Work out the finished part from the listing and answer in its coordinate system (mm). A direction names the side the tool comes from. Give positions to 0.01 mm unless a question says otherwise; leave off trailing zeros. Write each loop counter-clockwise with the first axis right and the second up, starting at its lowest first coordinate (ties: lowest second). Pieces come first, ordered by that corner, then holes. Notation, with made-up numbers: (8.25, 19) - (50.25, 19) arc R18 cw to (50.25, 27) - close; hole circle Ø2 at (68.25, -7). An arc over 180 degrees is marked (long way). Write item = value, one per line.
Autodesk Inventor part; units mm, degrees
ref_plane "YZ Plane" through (0, 0, 0) normal (1, 0, 0) x (0, 1, 0)
ref_plane "XZ Plane" through (0, 0, 0) normal (0, 1, 0) x (-1, 0, 0)
ref_plane "XY Plane" through (0, 0, 0) normal (0, 0, 1) x (1, 0, 0)
sketch "Szkic2" plane through (0, 0, 0) normal (0, 1, 0) x (-1, 0, 0)
  line L0 (10, 40) -> (-10, 40)
  line L1 (-10, 40) -> (-10, -40)
  line L2 (-10, -40) -> (10, -40)
  line L3 (10, -40) -> (10, 40)
  line L4 (10, 40) -> (-10, -40) construction
  line L5 (-10, 40) -> (10, -40) construction
  line L6 (8.6, 38.6) -> (-8.6, 38.6)
  line L7 (-8.6, 38.6) -> (-8.6, -38.6)
  line L8 (-8.6, -38.6) -> (8.6, -38.6)
  line L9 (8.6, -38.6) -> (8.6, 38.6)
  line L10 (8.6, 38.6) -> (-8.6, -38.6) construction
  line L11 (-8.6, 38.6) -> (8.6, -38.6) construction
  point P0 (0, 0)
  point P1 (0, -40)
  dimension "d14" = 20
  dimension "d15" = 80
  dimension "d16" = 1.4
  dimension "d17" = 1.4
extrude "Wyciągnięcie proste2" add sketch "Szkic2" along normal blind 500
sketch "Szkic3" plane through (-10, 0, -40) normal (-1, 0, 0) x (0, 0, 1)
  circle A0 centre (40, 229) radius 2.25
  circle A1 centre (40, 271) radius 2.25
  line L0 (0, 0) -> (0, 500)
  line L1 (0, 500) -> (80, 500)
  point P0 (40, 0)
  point P1 (40, 250)
  point P2 (40, 500)
  dimension "d20" = 4.5
  dimension "d21" = 4.5
  dimension "d22" = 21
  dimension "d23" = 21
  dimension "d24" = 40
  dimension "d25" = 40
  dimension "d26" = 40
  dimension "d27" = 250
extrude "Wyciągnięcie proste3" cut sketch "Szkic3" against normal blind 20
sketch "Szkic4" plane through (-10, 0, -40) normal (-1, 0, 0) x (0, 0, 1)
  point P0 (40, 0)
sketch "Szkic5" plane through (10, 0, 40) normal (1, 0, 0) x (0, 0, -1)
  point P0 (40, 0)
sketch "Szkic6" plane through (10, 0, 40) normal (1, 0, 0) x (0, 0, -1)
  point P0 (40, 0)
sketch "Szkic7" plane through (10, 0, 40) normal (1, 0, 0) x (0, 0, -1)
  line L0 (80, 0) -> (80, 500)
  line L1 (80, 250) -> (0, 250)
  line L2 (1.4, 0) -> (1.4, 500)
  line L3 (80, 250) -> (160, 250) construction
  line L4 (50, 355) -> (30, 355)
  line L5 (30, 355) -> (30, 325)
  line L6 (30, 325) -> (50, 325)
  line L7 (50, 325) -> (50, 355)
  line L8 (50, 355) -> (30, 325) construction
  line L9 (30, 355) -> (50, 325) construction
  line L10 (50, 145) -> (30, 145)
  line L11 (30, 145) -> (30, 175)
  line L12 (30, 175) -> (50, 175)
  line L13 (50, 175) -> (50, 145)
  point P0 (40, 0)
  point P1 (40, 340)
  dimension "d30" = 80
  dimension "d31" = 180
  dimension "d32" = 20
  dimension "d33" = 30
  dimension "d34" = 90
  dimension "d35" = 40
extrude "Wyciągnięcie proste4" cut sketch "Szkic7" against normal blind 1.4
sketch "Szkic8" plane through (-10, 0, -40) normal (-1, 0, 0) x (0, 0, 1)
  line L0 (0, 0) -> (0, 500)
  line L1 (0, 250) -> (80, 250)
  line L2 (80, 0) -> (80, 500)
  line L3 (0, 250) -> (80, 250) construction
  circle A0 centre (40, 40) radius 10
  line L4 (0, 0) -> (80, 0)
  circle A1 centre (40, 460) radius 10
  point P0 (40, 0)
  point P1 (40, 0)
  dimension "d38" = 80
  dimension "d39" = 0
  dimension "d40" = 20
  dimension "d41" = 40
  dimension "d42" = 40
extrude "Wyciągnięcie proste5" cut sketch "Szkic8" against normal blind 1.4 contours A0 | A1
properties part number "belka" material "Aluminium 6061"
1. Find section A-A, the plane z = 31. Give the vertices of the cut face in (x, y).
Solution:
outline = (-10, 0) - (-8.6, 0) - (-8.6, 500) - (-10, 500) - close; (8.6, 0) - (10, 0) - (10, 500) - (8.6, 500) - close
2. A tool of negligible diameter and unlimited length cuts with its end or side. For faces 4 (the flat face through (9, 500, 6)), 5 (the cylindrical face through (-9.31, 469.915, -1.302)), 6 (the flat face through (8.6, 246, 1)), from which of +Z, -Z, +X, -X, +Y, -Y can it reach the whole face along a straight path? Write none if from no direction.
Solution:
face_4 = +Z, -Z, +X, -X, +Y
face_5 = -X
face_6 = +Y, -Y
3. Find section C-C, the plane y = 262. Give the vertices of the cut face in (x, z).
Solution:
outline = (-10, -40) - (10, -40) - (10, 40) - (-10, 40) - close; hole (-8.6, -38.6) - (8.6, -38.6) - (8.6, 38.6) - (-8.6, 38.6) - close
4. Find section B-B, the plane x = -0.75. Give the vertices of the cut face in (y, z), then the cut area to 3 significant figures.
Solution:
outline = (0, -40) - (500, -40) - (500, -38.6) - (0, -38.6) - close; (0, 38.6) - (500, 38.6) - (500, 40) - (0, 40) - close
area = 1,400 mm^2
5. Find section D-D, the plane y = 460. Give the vertices of the cut face in (x, z), then the cut area to 3 significant figures.
Solution:
outline = (-10, -40) - (10, -40) - (10, 40) - (-10, 40) - (-10, 10) - (-8.6, 10) - (-8.6, 38.6) - (8.6, 38.6) - (8.6, -38.6) - (-8.6, -38.6) - (-8.6, -10) - (-10, -10) - close
area = 244 mm^2
6. For a pull along Z with two mould halves and no side action, classify faces 1 (the flat face through (0, 246, -40)), 2 (the cylindrical face through (-9.31, 30.24, -2.17)), 3 (the flat face through (9, 0, 6)) as pulls with the +Z half, pulls with the -Z half, needs draft (parallel to the pull), parting line crosses it, or undercut.
Solution:
face_1 = pulls with the -Z half
face_2 = undercut
face_3 = needs draft
7. Given pin 1 (3.5 mm diameter, centred on y = 229, z = 0, fed in from -X), flat-ended and moving along its own axis, determine where the tip first touches the part or whether it passes through.
Solution:
pin_1 = through
8. Straight lines are drawn through the part: line 1 (Y direction, x = -9.15, z = 0); line 2 (Y direction, x = 9, z = 0); line 3 (X direction, y = 67.5, z = -33). For each, find the intervals that lie inside material, in ascending order.
Solution:
line_1 = 0 to 30, 50 to 226.75, 231.25 to 268.75, 273.25 to 450, 470 to 500
line_2 = 0 to 145, 175 to 226.75, 231.25 to 268.75, 273.25 to 325, 355 to 500
line_3 = -10 to -8.6, 8.6 to 10
